The listing builds one solid part. Answer for the finished solid, in the listing's coordinates (mm). Round coordinates to 2 decimals unless told otherwise and drop trailing zeros. Loops run counter-clockwise (first coordinate to the right, second up) from the corner with the lowest first, then second, coordinate; pieces in that order, holes last. Notation, with made-up numbers: (69.5, 64) -> (120.5, 64) arc R26 ccw to (120.5, 91) -> close; hole circle Ø8 at (-28, 88.25). An arc over 180 degrees is marked (long way). Write each question's results on one line, items separated by ' | '. Start each with the question number.
(1) Flat-ended cylindrical pins translate along their axes: pin 1 (5 mm diameter, centred on x = 5.5, z = -11, fed in from -Y); pin 2 (10 mm diameter, centred on x = -12.5, y = -1, fed in from +Z); pin 3 (3 mm diameter, centred on x = -15, y = 11.5, fed in from -Z). Find the tip coordinate at first contact, or state that the pin passes through.
(2) The part is cut by section A-A (x = -5.5). Determine the outline of the cut face in (y, z) (3 decimals).
(3) Straight lines are drawn through the part: probe 1 along Y at (x, z) = (-11.5, -6.35) (3 decimals); probe 2 along X at (y, z) = (-15.5, 1); probe 3 along X at (y, z) = (-10.5, -3). For each, find the intervals that lie inside material, in ascending order.
(4) The part is cut by section B-B (x = 10). Determine the outline of the cut face in (y, z) (3 decimals).
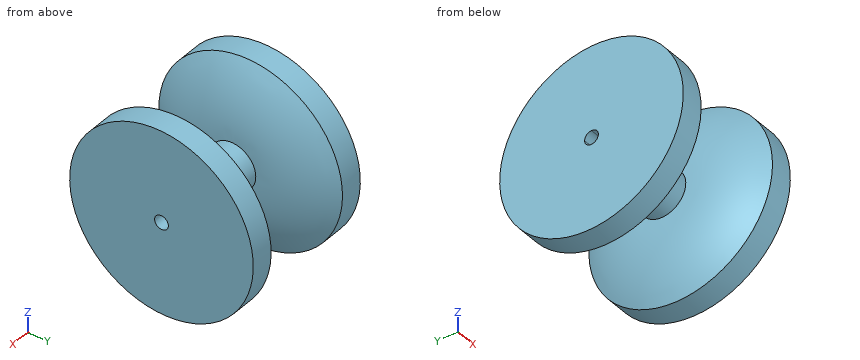
```python
from build123d import *

# Parameters (mm, degrees)
F3_DEPTH = 101.6


with BuildPart() as f1:
    # F0 (on Front) → F1 (revolve)
    with BuildSketch(Plane.XZ):
        with BuildLine():
            ThreePointArc((6.35, 19.05), (1.629305, 10.040232), (0, 0))
            Line((0, 0), (-12.7, 0))
            ThreePointArc((-12.7, 0), (-14.329305, 10.040232), (-19.05, 19.05))
            Line((-19.05, 19.05), (-25.4, 19.05))
            Line((-25.4, 19.05), (-25.4, -6.35))
            Line((-25.4, -6.35), (0, -6.35))
            Line((0, -6.35), (6.35, -6.35))
            Line((6.35, -6.35), (12.7, -6.35))
            Line((12.7, -6.35), (12.7, 19.05))
            Line((12.7, 19.05), (6.35, 19.05))
        make_face()
    revolve(axis=Axis((-6.35, 0, -6.35), (-1, 0, 0)))

    # F2 (on face) → F3 (cut)
    with BuildSketch(Plane.YZ.offset(12.7)):
        with BuildLine():
            Line((0, -6.35), (0, -4.445))
            ThreePointArc((0, -4.445), (-1.347038, -7.697038), (1.905, -6.35))
            Line((1.905, -6.35), (0, -6.35))
        make_face()
        with BuildLine():
            ThreePointArc((1.905, -6.35), (1.347038, -5.002962), (0, -4.445))
            Line((0, -4.445), (0, -6.35))
            Line((0, -6.35), (1.905, -6.35))
        make_face()
    extrude(amount=-F3_DEPTH, mode=Mode.SUBTRACT)


solid = f1.part
```
Checked values:
1) pin 1: stops at y = -25.3 | pin 2: stops at z = 16.77 | pin 3: stops at z = -24.54
2) outline: circle Ø12.7 at (0, -6.35); hole (0, -4.445) arc R1.905 ccw (long way) to (1.905, -6.35) arc R1.905 ccw to start
3) probe 1: y = -6.35 to -1.905, 1.905 to 6.35 | probe 2: x = -25.4 to -14.59, 1.89 to 12.7 | probe 3: x = -25.4 to -13.05, 0.35 to 12.7
4) outline: circle Ø50.8 at (0, -6.35); hole (0, -4.445) arc R1.905 ccw (long way) to (1.905, -6.35) arc R1.905 ccw to start
